Autodesk Inventor part; units mm, degrees
ref_plane "YZ Plane" through (0, 0, 0) normal (1, 0, 0) x (0, 1, 0)
ref_plane "XZ Plane" through (0, 0, 0) normal (0, 1, 0) x (-1, 0, 0)
ref_plane "XY Plane" through (0, 0, 0) normal (0, 0, 1) x (1, 0, 0)
sketch "Sketch1" plane through (0, 0, 0) normal (0, 0, 1) x (1, 0, 0)
  line L0 (0, 0) -> (220, 0)
  line L1 (220, 0) -> (220, 170)
  line L2 (220, 170) -> (0, 170)
  line L3 (0, 170) -> (0, 0)
  dimension "d0" = 220
  dimension "d1" = 170
extrude "Extrusion1" add sketch "Sketch1" along normal blind 100
sketch "Sketch2" plane through (0, 0, 0) normal (0, 0, 1) x (1, 0, 0)
  line L0 (5, 5) -> (215, 5)
  line L1 (215, 5) -> (215, 245)
  line L2 (215, 245) -> (5, 245)
  line L3 (5, 245) -> (5, 5)
  point P0 (0, 0)
  dimension "d4" = 210
  dimension "d5" = 240
  dimension "d8" = 5
  dimension "d13" = 5
extrude "Extrusion2" cut sketch "Sketch2" along normal blind 95
sketch "Sketch3" plane through (220, 0, 0) normal (1, 0, 0) x (0, 0, -1)
  circle A0 centre (-23.8569, 150) radius 15
  line L0 (0, 170) -> (-100, 170)
  point P0 (0, 0)
  dimension "d9" = 30
  dimension "d10" = 20
extrude "Extrusion3" cut sketch "Sketch3" against normal blind 45
sketch "Sketch4" plane through (0, 0, 0) normal (-1, 0, 0) x (0, 0, 1)
  circle A0 centre (73.7116, 232.2043) radius 14.7089
  point P0 (0, 0)
extrude "Extrusion4" [suppressed]
sketch "Sketch5" plane through (0, 0, 95) normal (0, 0, -1) x (-1, 0, 0)
  line L0 (-215, 170) -> (-5, 170)
  line L1 (-117.8578, 170) -> (-111.2412, 170)
  line L2 (-111.2412, 170) -> (-111.2412, 129.5746)
  line L3 (-111.2412, 129.5746) -> (-117.8578, 129.5746)
  line L4 (-117.8578, 129.5746) -> (-117.8578, 170)
  point P0 (0, 0)
extrude "Extrusion5" add sketch "Sketch5" along normal blind 35
properties part number "corpo"
Geometry: final body of the model. Coordinates: model frame, mm. A direction names the side the tool comes from. Round coordinates to 2 decimals unless told otherwise and drop trailing zeros. Write each loop counter-clockwise with the first axis right and the second up, starting at its lowest first coordinate (ties: lowest second). Pieces come first, ordered by that corner, then holes.
Item 1: Section query D-D (z = 53.5). Return loops of the section in (x, y).
Item 2: Mould query, pull axis X, two halves, no side actions, for faces 1 (the face through (5, 89, 47)), 2 (the face through (0, 86, 49)), 3 (the face through (220, 84, 49)), 4 (the face through (108, 0, 49)). Classes: +X half, -X half, draft (parallel to the pull), parting line (faces both ways), or undercut.
Item 3: Material intervals for L1, parallel to X at y = 150, z = 78; L2, parallel to X at y = 60, z = 41; L3, parallel to Y at x = 80.5, z = 47.5, sorted ascending.
Item 4: Section query C-C (y = 105). Return loops of the section in (x, z).
Item 5: Section query B-B (z = 89). Return loops of the section in (x, y).
Item 6: Pin query (flat end, axial travel): P1, Ø2, axis at x = 93.5, z = 21.5, coming from the -Y side; P2, Ø12, axis at x = 132.5, y = 33, coming from the -Z side; P3, Ø12, axis at x = 101, z = 44, coming from the +Y side; P4, Ø18, axis at y = 150, z = 23.86, coming from the +X side. Return the tip coordinate at first contact, or that it passes through.
Item 7: Section query A-A (y = 150). Return loops of the section in (x, z), plus the area to 3 significant figures.
Item 8: Set-up query: faces 5 (the face through (115, 129.575, 78)), 6 (the face through (217.54, 136.69, 16.94)), 7 (the face through (115, 150, 60)). Return all of +Z, -Z, +X, -X, +Y, -Y with unobstructed straight access to the full face (end or side cutting, diameter ignored); none if empty.
Completed:
1. outline: (0, 0) - (220, 0) - (220, 170) - (215, 170) - (215, 5) - (5, 5) - (5, 170) - (0, 170) - close
2. face 1: undercut
2. face 2: -X half
2. face 3: +X half
2. face 4: draft
3. L1: x = 0 to 5, 111.24 to 117.86, 215 to 220
3. L2: x = 0 to 5, 215 to 220
3. L3: y = 0 to 5
4. outline: (0, 0) - (5, 0) - (5, 95) - (215, 95) - (215, 0) - (220, 0) - (220, 100) - (0, 100) - close
5. outline: (0, 0) - (220, 0) - (220, 170) - (215, 170) - (215, 5) - (5, 5) - (5, 170) - (0, 170) - close; (111.24, 129.57) - (117.86, 129.57) - (117.86, 170) - (111.24, 170) - close
6. P1: stops at y = 0
6. P2: stops at z = 95
6. P3: stops at y = 5
6. P4: stops at x = 5
7. outline: (0, 0) - (5, 0) - (5, 95) - (111.24, 95) - (111.24, 60) - (117.86, 60) - (117.86, 95) - (215, 95) - (215, 38.86) - (220, 38.86) - (220, 100) - (0, 100) - close; (215, 0) - (220, 0) - (220, 8.86) - (215, 8.86) - close
7. area: 2,130 mm2
8. face 5: -Z
8. face 6: +X
8. face 7: -Z, +Y
